```python
from build123d import *

# Parameters (mm, degrees)
F0_R          = 25.5
F1_DEPTH      = 5.08
F3_R          = 28
F3_R_2        = 23.5
F4_DEPTH      = 1.5875
F5_DEPTH      = 1.5875
F5_DEPTH_BACK = 3.175
F6_DEPTH      = 1.5875
F9_R          = 24.5
F10_DEPTH     = 2.5
F11_R         = 1.27


# Not quite as in the source:
# - a fillet or chamfer that OpenCascade refuses, or shapes differently, is made with other operations: its cross-section is extruded or revolved along the edge and cut away or added


with BuildPart() as f1:
    # F0 (on Front) → F1 (new body)
    with BuildSketch(Plane.XZ):
        Circle(F0_R)
        with BuildLine():
            ThreePointArc((20.0593759089, -12.2421990731), (0, -23.5), (-20.0593759089, -12.2421990731))
            Line((-20.0593759089, -12.2421990731), (-15.990073811, -8.7466746798))
            Line((-15.990073811, -8.7466746798), (-18.1416651056, -6.2419074449))
            Line((-18.1416651056, -6.2419074449), (-21.61384866, -9.2245079057))
            ThreePointArc((-21.61384866, -9.2245079057), (0, 23.5), (21.61384866, -9.2245079057))
            Line((21.61384866, -9.2245079057), (18.1416651056, -6.2419074449))
            Line((18.1416651056, -6.2419074449), (15.990073811, -8.7466746798))
            Line((15.990073811, -8.7466746798), (20.0593759089, -12.2421990731))
        make_face(mode=Mode.SUBTRACT)
    extrude(amount=F1_DEPTH)

    # F3 (on face) → F4 (join)
    with BuildSketch(Plane.XZ.offset(5.08)):
        Circle(F3_R)
        Circle(F3_R_2, mode=Mode.SUBTRACT)
    extrude(amount=F4_DEPTH)

    # F2 (on face) → F5 (cut, two sides)
    with BuildSketch(Plane.XZ.offset(5.08)) as f5_sk:
        with BuildLine():
            Line((20, -14.7076810144), (-20, -14.7076810144))
            ThreePointArc((-20, -14.7076810144), (0, -24.8257100769), (20, -14.7076810144))
        make_face()
    extrude(amount=-F5_DEPTH, mode=Mode.SUBTRACT)
    extrude(f5_sk.sketch, amount=F5_DEPTH_BACK, mode=Mode.SUBTRACT)

    # F6 (cut): faces of the model
    f6_faces = [f1.faces().sort_by_distance(p)[0] for p in [
        (18.9429993018, -5.08, -9.163640961),
        (-18.9429993018, -5.08, -9.163640961),
    ]]
    extrude(f6_faces, amount=-F6_DEPTH, mode=Mode.SUBTRACT)

    # F7: chamfer of 1.5875 on 1 edges, made by hand

    # F7_s1 → F7_t2 (revolve, cut)
    with BuildSketch(Plane.XY):
        Polygon((26.4125, -5.08), (28, -6.6675), (28, -5.08), align=None)
    revolve(axis=Axis((0, -5.08, 0), (0, -1, 0)), mode=Mode.SUBTRACT)

    # F8: fillet of radius 5.08 on 1 edges, made by hand

    # F8_s1 → F8_t2 (revolve, cut)
    with BuildSketch(Plane.XY):
        with BuildLine():
            ThreePointArc((25.5, -5.08), (26.6871185711, -5.586485263), (27.7082857935, -6.3757857935))
            Line((27.7082857935, -6.3757857935), (26.4125, -5.08))
            Line((26.4125, -5.08), (25.5, -5.08))
        make_face()
    revolve(axis=Axis((0, -5.08, 0), (0, -1, 0)), mode=Mode.SUBTRACT)

    # F9 (on face) → F10 (cut)
    with BuildSketch(Plane.XZ.offset(6.6675)):
        Circle(F9_R)
    extrude(amount=-F10_DEPTH, mode=Mode.SUBTRACT)

    # F11
    f11_edges = [f1.edges().sort_by_distance(p)[0] for p in [
        (-15.990074, -1.74625, -8.746675),
        (-18.141665, -1.74625, -6.241907),
        (15.990074, -1.74625, -8.746675),
        (18.141665, -1.74625, -6.241907),
    ]]
    fillet(f11_edges, radius=F11_R)


solid = f1.part
```
CAD build for the part. Positions are in the model's coordinates, mm. A direction names the side the tool comes from. Coordinates: 2 decimals unless noted, no trailing zeros. Loops run counter-clockwise (first coordinate to the right, second up) from the corner with the lowest first, then second, coordinate; pieces in that order, holes last. Notation, with made-up numbers: (43, 65.5) - (49, 65.5) arc R31 ccw to (49, 104.5) - close; hole circle Ø4 at (-24.75, -12.75). An arc over 180 degrees is marked (long way). Use CSV: the item, a comma, the result in double quotes. Start each with the question number.
Q1. 3-axis set-ups, long thin cutter, end or side, ignore diameter. For faces 1 (the flat face through (18.485, -1.722, -10.89)), 2 (the flat face through (-17, 0, -9)), 3 (the flat face through (19, -3.492, -9)): which of +Z, -Z, +X, -X, +Y, -Y reach the whole face in a straight line?
Q2. Drop flat-ended pins along their axis: P1, Ø5, axis at x = 8.5, z = -19.5, coming from the -Y side; P2, Ø1.5, axis at x = -15, y = -5, coming from the -Z side; P3, Ø4, axis at x = -6.5, y = -4.5, coming from the +Z side; P4, Ø19.5, axis at x = 1.5, z = -2, coming from the -Y side. Give the stop position or say it passes through.
Q3. Cut at B-B, the plane z = 0. List the corners of the cut face in (x, y), then the cut area to 3 significant figures.
Q4. Probe probe 1 along Z at (x, y) = (0, -3.25); probe 2 along X at (y, z) = (-1, 6); probe 3 along Z at (x, y) = (-13, -6). List the from-to ranges inside material, lowest first. Write a range as from..to.
Q5. Two-plate mould, pull along Z, no slides. Class faces 4 (the cylindrical face through (-16.514, -1.771, -8.693)), 5 (the cylindrical face through (-5.5, -2.5, -24.9)), 6 (the flat face through (0, -6.668, 25)), 7 (the flat face through (-2, -3.492, -24)): +Z half, -Z half, draft (parallel to the pull), parting line (faces both ways), or undercut.
Q6. Cut at A-A, the plane x = 0. List the corners of the cut face in (y, z), then the cut area to 3 significant figures.
Here are the results:
1,face 1,"+Y, -Y"
1,face 2,"+Z, -Z, +X, -X, +Y"
1,face 3,"-Y"
2,P1,"y = -3.49"
2,P2,"z = -22.47"
2,P3,"z = 27.11"
2,P4,"through"
3,outline,"(-28, -6.67) - (-24.5, -6.67) - (-24.5, -4.17) - (-23.5, -4.17) - (-23.5, 0) - (-25.5, 0) - (-25.5, -5.08) arc R5.08 ccw to (-27.71, -6.38) - close; (23.5, -4.17) - (24.5, -4.17) - (24.5, -6.67) - (28, -6.67) - (27.71, -6.38) arc R5.08 ccw to (25.5, -5.08) - (25.5, 0) - (23.5, 0) - close"
3,area,"26.5 mm2"
4,probe 1,"-25.5..-23.5, 23.5..25.5"
4,probe 2,"-24.78..-22.72, 22.72..24.78"
4,probe 3,"-23.99..-21.15, 20.77..23.99"
5,face 4,"undercut"
5,face 5,"parting line"
5,face 6,"draft"
5,face 7,"undercut"
6,outline,"(-6.67, -28) - (-6.38, -27.71) arc R5.08 ccw to (-5.08, -25.5) - (0, -25.5) - (0, -23.5) - (-3.49, -23.5) - (-3.49, -24.83) - (-6.67, -24.83) - close; (-6.67, 24.5) - (-4.17, 24.5) - (-4.17, 23.5) - (0, 23.5) - (0, 25.5) - (-5.08, 25.5) arc R5.08 ccw to (-6.38, 27.71) - (-6.67, 28) - close"
6,area,"24.8 mm2"
